Source: CAD feature listing. Evaluate the final solid. Frame: model axes, mm. Face numbers are marked on the shaded views. Round coordinates to 2 decimals unless told otherwise and drop trailing zeros. Order: outer loops, then holes, each group sorted by start corner. A loop starts at its lowest first (then second) coordinate and runs counter-clockwise, first axis right, second up. Notation, with made-up numbers: (42.25, 11) -> (82.25, 11) arc R19 ccw to (82.25, 22) -> close; hole circle Ø4 at (20.25, 85.5). An arc over 180 degrees is marked (long way). One line per item, written item: value. Start each with the question number.
1) Section C-C (z = 55.5). Return the cut outline in (x, y).
2) Section D-D (x = -0.5). Return the cut outline in (y, z).
3) Section B-B (x = 9.75). Return the cut outline in (y, z), and give its area (3 significant figures).
4) Pin query (flat end, axial travel): P1, Ø1.5, axis at y = 1, z = -11.5, coming from the +X side; P2, Ø16, axis at y = 0, z = 24, coming from the -X side. Return the tip coordinate at first contact, or that it passes through.
5) Ray query, L1, parallel to Z at x = -0.5, y = 0; L2, parallel to Z at x = 3.5, y = -3; L3, parallel to Y at x = 2.75, z = -21. Return the intervals inside material, ascending.
6) Section A-A (y = 0). Return the cut outline in (x, z).
7) Mould query, pull axis Z, two halves, no side actions, for the marked faces 1, 2 and 3. Classes: pulls with the +Z half, pulls with the -Z half, needs draft (parallel to the pull), parting line crosses it, or undercut.
```python
from build123d import *

# Parameters (mm, degrees)
F1_DEPTH = 15.5
F2_R     = 6.5
F2_R_2   = 10
F2_R_3   = 8.5
F3_DEPTH = 28.001


with BuildPart() as f1:
    # F0 (on Front) → F1 (new body, symmetric)
    with BuildSketch(Plane.XZ):
        Polygon((14, 13), (14, 77), (-14, 77), (-14, -77), (14, -77), (14, -23), (8, -23), (8, 13), align=None)
    extrude(amount=F1_DEPTH, both=True)

    # F2 (on face) → F3 (cut, through all)
    with BuildSketch(Plane(origin=(-14, 0, 0), x_dir=(0, -1, 0), z_dir=(-1, 0, 0))):
        with Locations((0, 55.5)):
            Circle(F2_R)
        with Locations((0, 24)):
            Circle(F2_R_2)
        with Locations((0, -1)):
            Circle(F2_R_3)
        with Locations((0, -21)):
            Circle(F2_R)
        with Locations((0, -55.5)):
            Circle(F2_R)
    extrude(amount=-F3_DEPTH, mode=Mode.SUBTRACT)


solid = f1.part
```
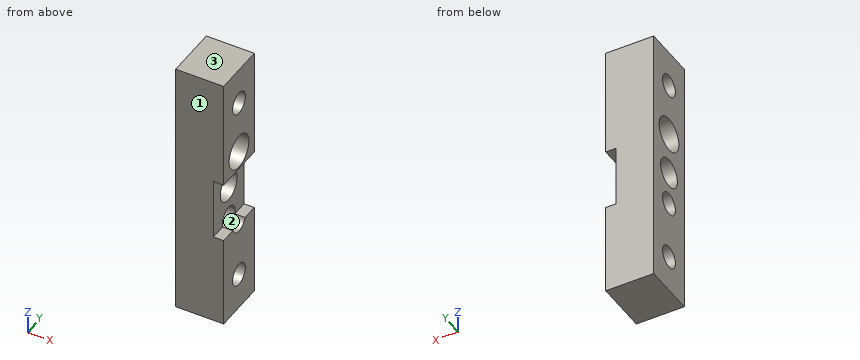
Findings:
1. outline: (-14, -15.5) -> (14, -15.5) -> (14, -6.5) -> (-14, -6.5) -> close; (-14, 6.5) -> (14, 6.5) -> (14, 15.5) -> (-14, 15.5) -> close
2. outline: (-15.5, -77) -> (15.5, -77) -> (15.5, 77) -> (-15.5, 77) -> close; hole circle Ø20 at (0, 24); hole circle Ø17 at (0, -1); hole circle Ø13 at (0, -55.5); hole circle Ø13 at (0, -21); hole circle Ø13 at (0, 55.5)
3. outline: (-15.5, -77) -> (15.5, -77) -> (15.5, -23) -> (6.18, -23) arc R6.5 cw to (-6.18, -23) -> (-15.5, -23) -> close; (-15.5, 13) -> (15.5, 13) -> (15.5, 77) -> (-15.5, 77) -> close; hole circle Ø20 at (0, 24); hole circle Ø13 at (0, -55.5); hole circle Ø13 at (0, 55.5)
3. area: 3,040 mm2
4. P1: x = 8
4. P2: through
5. L1: -77 to -62, -49 to -27.5, -14.5 to -9.5, 7.5 to 14, 34 to 49, 62 to 77
5. L2: -77 to -61.27, -49.73 to -26.77, -15.23 to -8.95, 6.95 to 14.46, 33.54 to 49.73, 61.27 to 77
5. L3: -15.5 to -6.5, 6.5 to 15.5
6. outline: (-14, -77) -> (14, -77) -> (14, -62) -> (-14, -62) -> close; (-14, -49) -> (14, -49) -> (14, -27.5) -> (-14, -27.5) -> close; (-14, -14.5) -> (8, -14.5) -> (8, -9.5) -> (-14, -9.5) -> close; (-14, 7.5) -> (8, 7.5) -> (8, 13) -> (14, 13) -> (14, 14) -> (-14, 14) -> close; (-14, 34) -> (14, 34) -> (14, 49) -> (-14, 49) -> close; (-14, 62) -> (14, 62) -> (14, 77) -> (-14, 77) -> close
7. face 1: needs draft
7. face 2: undercut
7. face 3: pulls with the +Z half
